Can you work these out from the drawing? Everything is in mm from the part's minimum corner. Round coordinates to 2 decimals unless told otherwise and drop trailing zeros. Write each loop counter-clockwise with the first axis right and the second up, starting at its lowest first coordinate (ties: lowest second). Pieces come first, ordered by that corner, then holes. Notation, with made-up numbers: (83, 61.25) - (108, 61.25) arc R17 ccw to (108, 82.25) - close; hole circle Ø7 at (31.5, -5). An arc over 180 degrees is marked (long way). One line per item, written item: value. Start each with the question number.
(1) I want a section at B-B on y = 2.3. List the corners of the cut face in (x, z) for me, plus the area to 3 significant figures.
(2) If I drill on L1, parallel to Z at x = 34, y = 3.35; L2, parallel to Z at x = 59, y = 0.8; L3, parallel to Z at x = 33, y = 3.95, over which ranges is the centre line in solid material (lowest first)? Write a range as from..to.
(3) I'm going to push a flat-ended pin straight in: pin 1 Ø2.5 at (x, y) = (12.5, 3) entering from -Z. Where does the tip first touch, or does it pass through?
(4) I want a section at A-A on x = 34. List the corners of the cut face in (y, z) for me.
(5) I want a section at C-C on z = 4.5. List the corners of the cut face in (x, y) for me.
(6) I want a section at D-D on x = 10.5. List the corners of the cut face in (y, z) for me.
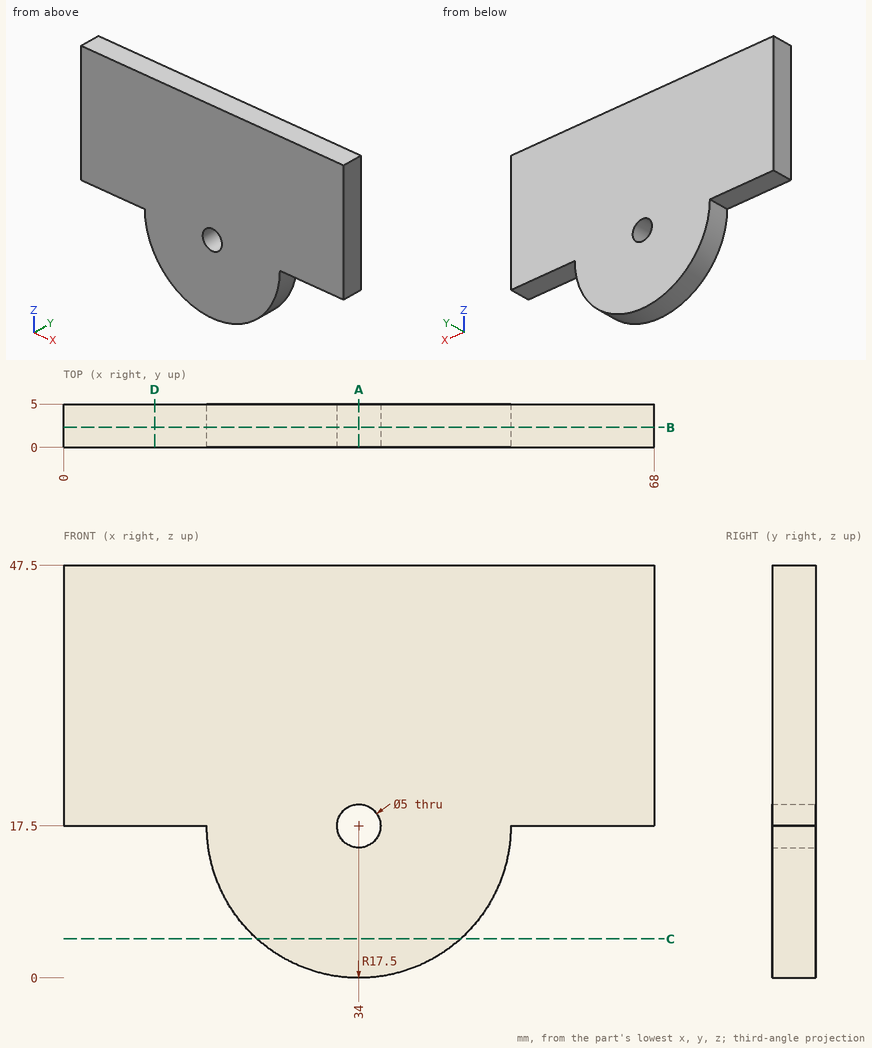
Established:
1. outline: (0, 17.5) - (16.5, 17.5) arc R17.5 ccw to (51.5, 17.5) - (68, 17.5) - (68, 47.5) - (0, 47.5) - close; hole circle Ø5 at (34, 17.5)
1. area: 2,500 mm2
2. L1: 0..15, 20..47.5
2. L2: 17.5..47.5
2. L3: 0.03..15.21, 19.79..47.5
3. pin 1: z = 17.5
4. outline: (0, 0) - (5, 0) - (5, 15) - (0, 15) - close; (0, 20) - (5, 20) - (5, 47.5) - (0, 47.5) - close
5. outline: (22.28, 0) - (45.72, 0) - (45.72, 5) - (22.28, 5) - close
6. outline: (0, 17.5) - (5, 17.5) - (5, 47.5) - (0, 47.5) - close
